```python
from build123d import *

# Parameters (mm, degrees)
F0_R     = 3.175
F1_DEPTH = 25.4
F2_DEPTH = 25.4


with BuildPart() as f1:
    # F0 (on Front) → F1 (new body)
    with BuildSketch(Plane.XZ):
        with BuildLine():
            ThreePointArc((-21.8341132764, 59.9675301176), (-18.9958831699, 53.1842614814), (-12.1726469476, 50.4435077562))
            ThreePointArc((-12.1726469476, 50.4435077562), (-5.5258446402, 53.2807602241), (-2.7841132764, 59.9675301176))
            ThreePointArc((-2.7841132764, 59.9675301176), (-2.7904513825, 60.3149502538), (-2.8094572661, 60.6619080307))
            ThreePointArc((-2.8094572661, 60.6619080307), (-12.6565334125, 69.4861920114), (-21.8341132764, 59.9675301176))
        make_face()
        with BuildLine():
            ThreePointArc((-9.1341132764, 59.9675301176), (-10.048023731, 57.7386068198), (-12.2636245001, 56.7928559971))
            ThreePointArc((-12.2636245001, 56.7928559971), (-14.5702028218, 62.1964534155), (-9.1341132764, 59.9675301176))
        make_face(mode=Mode.SUBTRACT)
        with BuildLine():
            ThreePointArc((-2.7841132764, 59.9675301176), (-5.5258446402, 53.2807602241), (-12.1726469476, 50.4435077562))
            Line((-12.1726469476, 50.4435077562), (-11.8086620269, 25.04090072))
            ThreePointArc((-11.8086620269, 25.04090072), (-2.4270394488, 22.1373657907), (3.4513160797, 14.2703273667))
            Line((3.4513160797, 14.2703273667), (-2.8094572661, 60.6619080307))
            ThreePointArc((-2.8094572661, 60.6619080307), (-2.7904513825, 60.3149502538), (-2.7841132764, 59.9675301176))
        make_face()
        with BuildLine():
            Line((-11.8086620269, 25.04090072), (-12.1726469476, 50.4435077562))
            ThreePointArc((-12.1726469476, 50.4435077562), (-18.9958831699, 53.1842614814), (-21.8341132764, 59.9675301176))
            Line((-21.8341132764, 59.9675301176), (-27.0492958066, 12.7388321873))
            ThreePointArc((-27.0492958066, 12.7388321873), (-21.5523049303, 21.5203861976), (-11.8086620269, 25.04090072))
        make_face()
        with Locations((-17.0401986688, 45.1469011605)):
            Circle(F0_R, mode=Mode.SUBTRACT)
        with BuildLine():
            ThreePointArc((3.4513160797, 14.2703273667), (-2.4270394488, 22.1373657907), (-11.8086620269, 25.04090072))
            Line((-11.8086620269, 25.04090072), (-11.6267069219, 12.3422042381))
            ThreePointArc((-11.6267069219, 12.3422042381), (-9.3522948478, 11.428619663), (-8.4062181456, 9.1675301176))
            ThreePointArc((-8.4062181456, 9.1675301176), (-9.3361541153, 6.9224660873), (-11.5812181456, 5.9925301176))
            Line((-11.5812181456, 5.9925301176), (-11.5812181456, -6.7074698824))
            ThreePointArc((-11.5812181456, -6.7074698824), (-1.1742480118, -2.8204053858), (4.1363360906, 6.9372579749))
            Line((4.1363360906, 6.9372579749), (4.2661999847, 8.232135226))
            Line((4.2661999847, 8.232135226), (3.4513160797, 14.2703273667))
        make_face()
        with BuildLine():
            Line((-11.6267069219, 12.3422042381), (-11.8086620269, 25.04090072))
            ThreePointArc((-11.8086620269, 25.04090072), (-21.5523049303, 21.5203861976), (-27.0492958066, 12.7388321873))
            Line((-27.0492958066, 12.7388321873), (-27.4558348468, 9.0572142544))
            Line((-27.4558348468, 9.0572142544), (-27.1667644493, 6.1498536246))
            ThreePointArc((-27.1667644493, 6.1498536246), (-21.6834458869, -3.0783107953), (-11.5812181456, -6.7074698824))
            Line((-11.5812181456, -6.7074698824), (-11.5812181456, 5.9925301176))
            ThreePointArc((-11.5812181456, 5.9925301176), (-14.7561366747, 9.1447851458), (-11.6267069219, 12.3422042381))
        make_face()
        with BuildLine():
            ThreePointArc((4.2937818544, 9.1675301176), (4.0817494185, 11.7534674886), (3.4513160797, 14.2703273667))
            Line((3.4513160797, 14.2703273667), (4.2661999847, 8.232135226))
            ThreePointArc((4.2661999847, 8.232135226), (4.2868848888, 8.6996293902), (4.2937818544, 9.1675301176))
        make_face()
        with BuildLine():
            Line((-27.4558348468, 9.0572142544), (-27.0492958066, 12.7388321873))
            ThreePointArc((-27.0492958066, 12.7388321873), (-27.3603087443, 10.9099206818), (-27.4558348468, 9.0572142544))
        make_face()
        with BuildLine():
            ThreePointArc((4.1363360906, 6.9372579749), (4.2145422634, 7.5833653216), (4.2661999847, 8.232135226))
            Line((4.2661999847, 8.232135226), (4.1363360906, 6.9372579749))
        make_face()
        with BuildLine():
            Line((-27.1667644493, 6.1498536246), (-27.4558348468, 9.0572142544))
            ThreePointArc((-27.4558348468, 9.0572142544), (-27.3783270751, 7.5968695977), (-27.1667644493, 6.1498536246))
        make_face()
        with BuildLine():
            ThreePointArc((4.1363360906, 6.9372579749), (-1.1742480118, -2.8204053858), (-11.5812181456, -6.7074698824))
            Line((-11.5812181456, -6.7074698824), (-11.5812181456, -44.8074698824))
            ThreePointArc((-11.5812181456, -44.8074698824), (-4.8460260548, -47.5972777916), (-2.0562181456, -54.3324698824))
            Line((-2.0562181456, -54.3324698824), (24.9312818544, -54.3324698824))
            ThreePointArc((24.9312818544, -54.3324698824), (27.3568713697, -48.6208370985), (33.1511871289, -46.3999952678))
            Line((33.1511871289, -46.3999952678), (7.3831695342, -45.4826240265))
            ThreePointArc((7.3831695342, -45.4826240265), (1.67659756, -42.7654990677), (-0.2444901556, -36.7441077228))
            Line((-0.2444901556, -36.7441077228), (4.1363360906, 6.9372579749))
        make_face()
        with BuildLine():
            Line((-11.5812181456, -44.8074698824), (-11.5812181456, -6.7074698824))
            ThreePointArc((-11.5812181456, -6.7074698824), (-21.6834458869, -3.0783107953), (-27.1667644493, 6.1498536246))
            Line((-27.1667644493, 6.1498536246), (-21.0594835033, -55.2748661943))
            ThreePointArc((-21.0594835033, -55.2748661943), (-18.6417404305, -47.9391413233), (-11.5812181456, -44.8074698824))
        make_face()
        with BuildLine():
            Line((-11.5812181456, -51.1574698824), (-11.5812181456, -44.8074698824))
            ThreePointArc((-11.5812181456, -44.8074698824), (-18.6417404305, -47.9391413233), (-21.0594835033, -55.2748661943))
            ThreePointArc((-21.0594835033, -55.2748661943), (-17.9745467047, -61.3929921673), (-11.5812181456, -63.8574698824))
            Line((-11.5812181456, -63.8574698824), (-10.9038745977, -63.8333556684))
            ThreePointArc((-10.9038745977, -63.8333556684), (-4.6106614141, -60.8237689706), (-2.0562181456, -54.3324698824))
            Line((-2.0562181456, -54.3324698824), (-8.4062181456, -54.3324698824))
            ThreePointArc((-8.4062181456, -54.3324698824), (-13.8262821759, -56.5775339127), (-11.5812181456, -51.1574698824))
        make_face()
        with BuildLine():
            Line((24.9312818544, -54.3324698824), (-2.0562181456, -54.3324698824))
            ThreePointArc((-2.0562181456, -54.3324698824), (-4.6106614141, -60.8237689706), (-10.9038745977, -63.8333556684))
            Line((-10.9038745977, -63.8333556684), (33.1511871289, -62.264944497))
            ThreePointArc((33.1511871289, -62.264944497), (27.3568713697, -60.0441026663), (24.9312818544, -54.3324698824))
        make_face()
        with BuildLine():
            Line((-10.9038745977, -63.8333556684), (-11.5812181456, -63.8574698824))
            ThreePointArc((-11.5812181456, -63.8574698824), (-11.2423318161, -63.8514394199), (-10.9038745977, -63.8333556684))
        make_face()
        with BuildLine():
            ThreePointArc((33.1511871289, -46.3999952678), (27.3568713697, -48.6208370985), (24.9312818544, -54.3324698824))
            ThreePointArc((24.9312818544, -54.3324698824), (27.3568713697, -60.0441026663), (33.1511871289, -62.264944497))
            ThreePointArc((33.1511871289, -62.264944497), (38.5804146383, -59.8443803671), (40.8062818544, -54.3324698824))
            ThreePointArc((40.8062818544, -54.3324698824), (38.5804146383, -48.8205593977), (33.1511871289, -46.3999952678))
        make_face()
        with BuildLine():
            ThreePointArc((36.0437818544, -54.3324698824), (32.8687818544, -57.5074698824), (29.6937818544, -54.3324698824))
            ThreePointArc((29.6937818544, -54.3324698824), (32.8687818544, -51.1574698824), (36.0437818544, -54.3324698824))
        make_face(mode=Mode.SUBTRACT)
    extrude(amount=F1_DEPTH)

    # F0 (on Front) → F2 (join)
    with BuildSketch(Plane.XZ):
        with BuildLine():
            ThreePointArc((-2.0562181456, -54.3324698824), (-4.8460260548, -47.5972777916), (-11.5812181456, -44.8074698824))
            Line((-11.5812181456, -44.8074698824), (-11.5812181456, -51.1574698824))
            ThreePointArc((-11.5812181456, -51.1574698824), (-9.3361541153, -52.0874058521), (-8.4062181456, -54.3324698824))
            Line((-8.4062181456, -54.3324698824), (-2.0562181456, -54.3324698824))
        make_face()
    extrude(amount=F2_DEPTH)


solid = f1.part
```
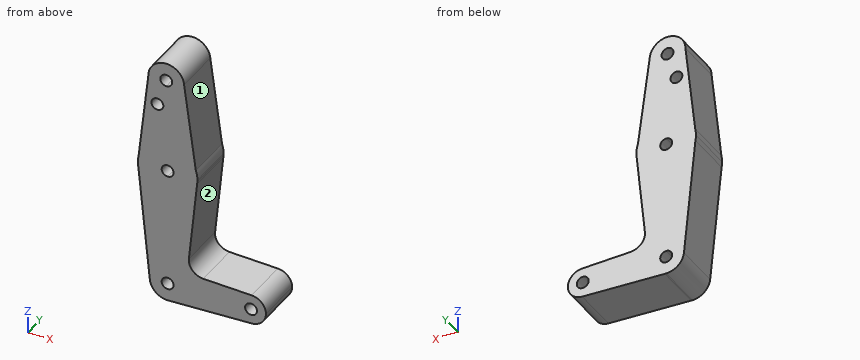
The listing builds one solid part. Answer for the finished solid, in the listing's coordinates (mm). Face numbers are marked on the shaded views. A direction names the side the tool comes from. Coordinates: 2 decimals unless noted, no trailing zeros. Loops run counter-clockwise (first coordinate to the right, second up) from the corner with the lowest first, then second, coordinate; pieces in that order, holes last. Notation, with made-up numbers: M 48.25,-2 L 96.25,-2 A23 cw 96.25,25 Z; hole C 58.5,64 d9. An arc over 180 degrees is marked long. Answer as CSV lines item,"result". Start each with the question number.
(1) The part is cut by section B-B (y = -5.5). State how many separate pieces and enclosed holes the cut face has, and give its area (3 significant figures).
(2) Given pin 1 (2 mm diameter, centred on y = -5.5, z = 22.5, fed in from +X); pin 2 (8.5 mm diameter, centred on x = 32.87, z = -54.33, fed in from -Y); pin 3 (1.5 mm diameter, centred on y = -17.5, z = -36, fed in from +X); pin 4 (5 mm diameter, centred on x = -17, y = -18, fed in from -Z), each flat-ended and moving along its own axis, determine where each tip first touches the part or whether it passes through.
(3) For the marked faces 1 and 2, determine the directions among +Z, -Z, +X, -X, +Y, -Y from which every point of the face is accessible in a straight line to the end or side of a thin tool.
(4) Find the intervals of material crossed by L1, parallel to X at y = -19.75, z = -55; L2, parallel to Z at x = 35, y = -12; L3, parallel to Z at x = -13.5, y = -20, in increasing order. Write a range as [from, to].
(5) The part is cut by section A-A (x = 2). Give the vertices of the cut face in (y, z).
(6) The part is cut by section C-C (z = -27.5). Give the vertices of the cut face in (x, y), and give its area (3 significant figures).
(7) The part is cut by section D-D (x = -18). Give the vertices of the cut face in (y, z).
Determined:
1,separate pieces,"1"
1,enclosed holes,"5"
1,area,"3,760 mm2"
2,pin 1,"x = 2.48"
2,pin 2,"y = -25.4"
2,pin 3,"x = -0.09"
2,pin 4,"z = -63.4"
3,face 1,"+Z, +X, +Y, -Y"
3,face 2,"+X, +Y, -Y"
4,L1,"[-21.09, -14.69], [-8.48, 29.76], [35.97, 40.78]"
4,L2,"[-61.98, -56.69], [-51.98, -46.69]"
4,L3,"[-63.66, -56.86], [-51.8, 6.64], [11.7, 57.02], [62.91, 69.42]"
5,outline,"M -25.4,-63.37 L 0,-63.37 L 0,-43.11 L -25.4,-43.11 Z; M -25.4,-14.36 L 0,-14.36 L 0,25.02 L -25.4,25.02 Z"
6,outline,"M -23.82,-25.4 L 0.68,-25.4 L 0.68,0 L -23.82,0 Z"
6,area,"622 mm2"
7,outline,"M -25.4,-61.37 L 0,-61.37 L 0,42.12 L -25.4,42.12 Z; M -25.4,48.17 L 0,48.17 L 0,67.61 L -25.4,67.61 Z"
